Drawing for the job (mm, zero at the part's lowest x, y, z). A direction names the side the tool comes from. Coordinates: 2 decimals unless noted, no trailing zeros. Order: outer loops, then holes, each group sorted by start corner. A loop starts at its lowest first (then second) coordinate and runs counter-clockwise, first axis right, second up.
1) Mould opens along Z. For the marked faces 4, 5 and 6 say: +Z half, -Z half, draft (parallel to the pull), parting line (faces both ways), or undercut.
2) Cut at A-A (y = 150). List the corners of the cut face in (x, z).
3) Cut at D-D (z = 200.5). List the corners of the cut face in (x, y).
4) Wall check: L1, parallel to Y at x = 78, z = 150; L2, parallel to X at y = 182, z = 283; L3, parallel to Z at x = 33.5, y = 185.5. Give the ranges that are in metal, low to high.
5) Pin check, flat tips, straight feed: pin 1 Ø4 at (x, y) = (32.5, 196) entering from +Z; pin 2 Ø1 at (y, z) = (62, 147) entering from -X; pin 3 Ø3 at (y, z) = (46.5, 235.5) entering from +X. Stop position of each tip, or through.
6) Cut at B-B (z = 150). List the corners of the cut face in (x, y), and give its area (3 significant figures).
7) Tool access for the marked faces 1, 2 and 3: list every direction of +Z, -Z, +X, -X, +Y, -Y with a clear straight run to the whole face (end or side of a thin tool).
8) Cut at C-C (x = 50.5). List the corners of the cut face in (y, z).
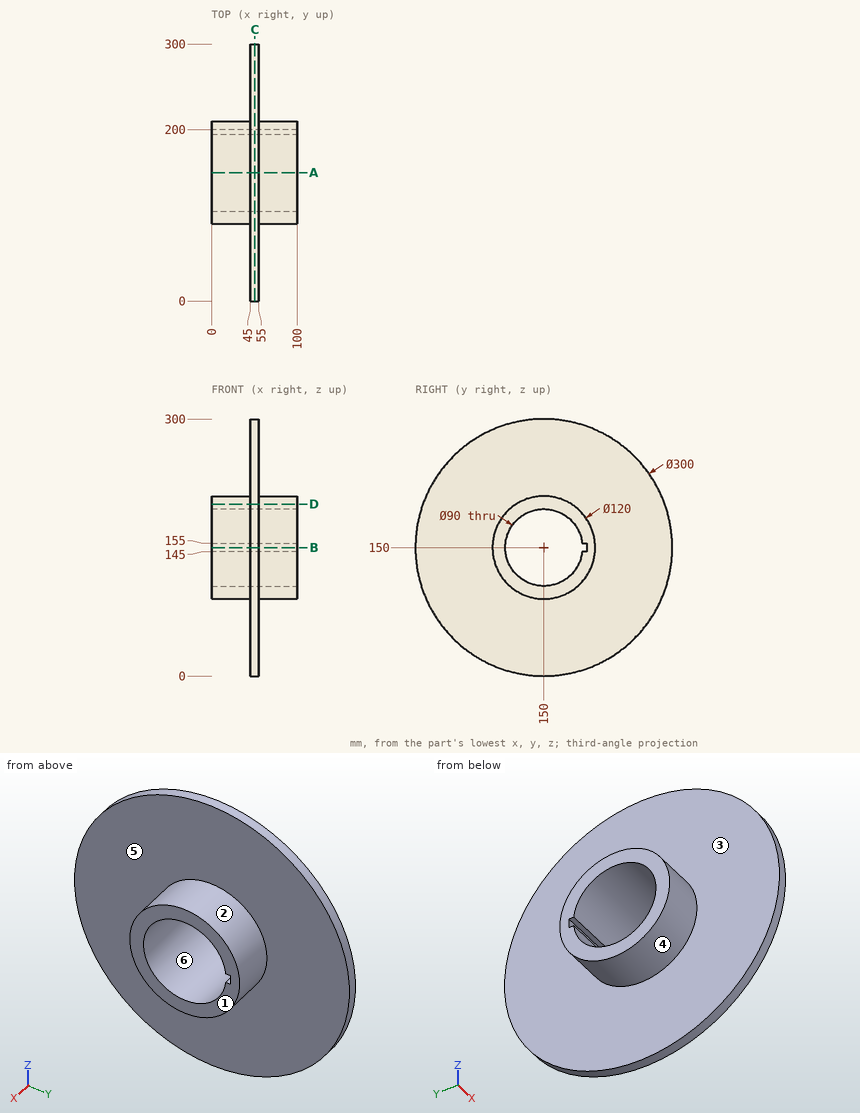
Geometry check:
1. face 4: parting line
1. face 5: draft
1. face 6: undercut
2. outline: (0, 90) - (45, 90) - (45, 0) - (55, 0) - (55, 90) - (100, 90) - (100, 105) - (0, 105) - close; (0, 195) - (100, 195) - (100, 210) - (55, 210) - (55, 300) - (45, 300) - (45, 210) - (0, 210) - close
3. outline: (0, 117.6) - (45, 117.6) - (45, 8.76) - (55, 8.76) - (55, 117.6) - (100, 117.6) - (100, 182.4) - (55, 182.4) - (55, 291.24) - (45, 291.24) - (45, 182.4) - (0, 182.4) - close
4. L1: y = 90 to 105, 200 to 210
4. L2: x = 45 to 55
4. L3: z = 101.63 to 122.35, 177.65 to 198.37
5. pin 1: stops at z = 190.79
5. pin 2: stops at x = 45
5. pin 3: stops at x = 55
6. outline: (0, 90) - (45, 90) - (45, 0) - (55, 0) - (55, 90) - (100, 90) - (100, 105) - (0, 105) - close; (0, 200) - (100, 200) - (100, 210) - (55, 210) - (55, 300) - (45, 300) - (45, 210) - (0, 210) - close
6. area: 4,300 mm2
7. face 1: +Z, -Z, +X, +Y, -Y
7. face 2: +X
7. face 3: -X
8. outline: circle Ø300 at (150, 150); hole (194.72, 145) - (200, 145) - (200, 155) - (194.72, 155) arc R45 ccw (long way) to start
